Part model, mm, in its own coordinate system. A direction names the side the tool comes from. Give positions to 0.01 mm unless a question says otherwise; leave off trailing zeros. Write each loop counter-clockwise with the first axis right and the second up, starting at its lowest first coordinate (ties: lowest second). Pieces come first, ordered by that corner, then holes. Notation, with made-up numbers: (-34, 89) - (5, 89) arc R10 ccw to (5, 106) - close; hole circle Ø4 at (-39.75, 24). An arc over 180 degrees is marked (long way). Answer in a Markdown table with one row per item. Add a question column.
1. Which spindle directions (+Z, -Z, +X, -X, +Y, -Y) get a long thin tool onto all of the face, cutting with end or side? Do faces 5 (the flat face through (14, -4, 1)), 6 (the flat face through (16, -4, 1)), 7 (the flat face through (30, 7, 8)), 8 (the flat face through (31, 11, 18)), 9 (the flat face through (14.8, 0, 10.8)). Say none if no direction does.
2. Band-saw the part on D-D on z = 3.75. Write the cut outline in (x, y).
3. Drop flat-ended pins along their axis: pin 1 Ø2 at (y, z) = (4.5, 18) entering from +X; pin 2 Ø5 at (y, z) = (9.5, 14) entering from -X; pin 3 Ø11 at (x, z) = (11.5, 14.5) entering from -Y; pin 4 Ø10 at (x, y) = (15, 4) entering from +Z. Give the stop position or say it passes through.
4. Band-saw the part on C-C on z = 17.25. Write the cut outline in (x, y), plus the area to 3 significant figures.
5. Band-saw the part on A-A on y = 0.75. Write the cut outline in (x, z).
6. Probe line 1 along X through (y, z) = (2.25, 1.75); line 2 along Y through (x, z) = (9, 7.5); line 3 along X through (y, z) = (4.75, 5.5). List the from-to ranges inside material, lowest first.
7. Pull direction Y, two halves, no side cores. Call faces 1 (the flat face through (31, 3, 18)), 2 (the flat face through (-3, 7, 11)), 3 (the flat face through (-2, 7, 13.5)), 4 (the flat face through (15, 17, 11)): released by +Y, released by -Y, zero draft, split by the parting line, or undercut.
8. Band-saw the part on B-B on x = 6. Write the cut outline in (y, z), plus the area to 3 significant figures.
```python
from build123d import *

# Parameters (mm, degrees)
SKETCH_1_W          = 36
SKETCH_1_H          = 20
SKETCH_1_W_2        = 30
SKETCH_1_H_2        = 14
EXTRUDE_2_DEPTH     = 22
SKETCH_2_W          = 9
SKETCH_2_H          = 14
EXTRUDE_3_DEPTH     = 4.5
SKETCH_4_W          = 2
SKETCH_4_H          = 2
EXTRUDE_4_DEPTH     = 2
CUT_EXTRUDE_1_REACH = 46.418
SKETCH_5_W          = 12
SKETCH_5_H          = 11
SKETCH_6_W          = 36
SKETCH_6_H          = 8
CUT_EXTRUDE_2_DEPTH = 8.5


with BuildPart() as part:
    # 스케치1 → 보스-돌출2 (new body)
    with BuildSketch(Plane.XY):
        with Locations((15, 7)):
            Rectangle(SKETCH_1_W, SKETCH_1_H)
        with Locations((15, 7)):
            Rectangle(SKETCH_1_W_2, SKETCH_1_H_2, mode=Mode.SUBTRACT)
    extrude(amount=EXTRUDE_2_DEPTH)

    # 스케치2 → 보스-돌출3 (add)
    with BuildSketch(Plane(origin=(0, 0, 0), x_dir=(-1, 0, 0), z_dir=(0, 0, -1))):
        with Locations((-15.5, 7)):
            Rectangle(SKETCH_2_W, SKETCH_2_H)
    extrude(amount=-EXTRUDE_3_DEPTH)

    # 스케치4 → 보스-돌출4 (add)
    with BuildSketch(Plane(origin=(0, 0, 0), x_dir=(-1, 0, 0), z_dir=(0, 0, -1))):
        with Locations((-15, -4)):
            Rectangle(SKETCH_4_W, SKETCH_4_H)
    extrude(amount=-EXTRUDE_4_DEPTH)

    # 스케치5 → 컷-돌출1 (cut, up to next)
    with BuildSketch(Plane.XZ.offset(3), mode=Mode.PRIVATE) as cut_extrude_1_sk1:
        with Locations((15, 16.5)):
            Rectangle(SKETCH_5_W, SKETCH_5_H)
    cut_extrude_1_tool1 = extrude(cut_extrude_1_sk1.sketch, amount=-CUT_EXTRUDE_1_REACH, mode=Mode.PRIVATE) & part.part
    add(cut_extrude_1_tool1.solids().sort_by_distance((15, -3, 16.5))[0], mode=Mode.SUBTRACT)

    # 스케치6 → 컷-돌출2 (cut)
    with BuildSketch(Plane.XY.offset(22)):
        with Locations((15, 7)):
            Rectangle(SKETCH_6_W, SKETCH_6_H)
    extrude(amount=-CUT_EXTRUDE_2_DEPTH, mode=Mode.SUBTRACT)


solid = part.part
```
Values:
| question | item | result |
|---|---|---|
| 1 | face 5 | +Z, -Z, -X, -Y |
| 1 | face 6 | +Z, -Z, +X, -Y |
| 1 | face 7 | +Z, -Z |
| 1 | face 8 | +Z, +X, -X |
| 1 | face 9 | +Z |
| 2 | outline | (-3, -3) - (33, -3) - (33, 17) - (-3, 17) - close; hole (0, 0) - (11, 0) - (11, 14) - (0, 14) - close; hole (20, 0) - (30, 0) - (30, 14) - (20, 14) - close |
| 3 | pin 1 | passes through |
| 3 | pin 2 | stops at x = -3 |
| 3 | pin 3 | stops at y = -3 |
| 3 | pin 4 | stops at z = 11 |
| 4 | outline | (-3, -3) - (9, -3) - (9, 0) - (0, 0) - (0, 3) - (-3, 3) - close; (-3, 11) - (0, 11) - (0, 14) - (30, 14) - (30, 11) - (33, 11) - (33, 17) - (-3, 17) - close; (21, -3) - (33, -3) - (33, 3) - (30, 3) - (30, 0) - (21, 0) - close |
| 4 | area | 216 mm² |
| 5 | outline | (-3, 0) - (0, 0) - (0, 22) - (-3, 22) - close; (11, 0) - (20, 0) - (20, 4.5) - (11, 4.5) - close; (30, 0) - (33, 0) - (33, 22) - (30, 22) - close |
| 6 | line 1 | x = -3 to 0, 11 to 20, 30 to 33 |
| 6 | line 2 | y = -3 to 0, 14 to 17 |
| 6 | line 3 | x = -3 to 0, 30 to 33 |
| 7 | face 1 | undercut |
| 7 | face 2 | zero draft |
| 7 | face 3 | undercut |
| 7 | face 4 | released by +Y |
| 8 | outline | (-3, 0) - (0, 0) - (0, 22) - (-3, 22) - close; (14, 0) - (17, 0) - (17, 22) - (14, 22) - close |
| 8 | area | 132 mm² |
